Model file for the job. Use its own axes, mm. Round coordinates to 2 decimals unless told otherwise and drop trailing zeros. Order: outer loops, then holes, each group sorted by start corner. A loop starts at its lowest first (then second) coordinate and runs counter-clockwise, first axis right, second up. Notation, with made-up numbers: (80.25, -8.75) - (112.25, -8.75) arc R20 cw to (112.25, 18.25) - close; hole circle Ø2 at (-30, 60.5). An arc over 180 degrees is marked (long way). Write item = value, one per line.
```python
from build123d import *

# Parameters (mm, degrees)
F1_DEPTH = 25.4


with BuildPart() as f1:
    # F0 (on Right) → F1 (new body)
    with BuildSketch(Plane.YZ):
        with BuildLine():
            ThreePointArc((-32.9688712955, -74.7904999055), (-16.4519134228, -59.7619169827), (0.0058700323, -74.8552786289))
            Line((0.0058700323, -74.8552786289), (0.610534451, 75.7063031197))
            Line((0.610534451, 75.7063031197), (-32.9688712955, 75.7063031197))
            Line((-32.9688712955, 75.7063031197), (-32.9688712955, -74.7904999055))
        make_face()
        with BuildLine():
            Line((-9.1503931598, -76.3168334961), (3.395e-07, -76.3168334961))
            Line((3.395e-07, -76.3168334961), (0.0058700323, -74.8552786289))
            ThreePointArc((0.0058700323, -74.8552786289), (-16.4519134228, -59.7619169827), (-32.9688712955, -74.7904999055))
            Line((-32.9688712955, -74.7904999055), (-32.9688712955, -76.3168334961))
            Line((-32.9688712955, -76.3168334961), (-23.8184777961, -76.3168334961))
            ThreePointArc((-23.8184777961, -76.3168334961), (-16.484435478, -68.982791178), (-9.1503931598, -76.3168334961))
        make_face()
        with BuildLine():
            Line((0.0058700323, -74.8552786289), (3.395e-07, -76.3168334961))
            Line((3.395e-07, -76.3168334961), (-9.1503931598, -76.3168334961))
            ThreePointArc((-9.1503931598, -76.3168334961), (-16.484435478, -83.6508758142), (-23.8184777961, -76.3168334961))
            Line((-23.8184777961, -76.3168334961), (-32.9688712955, -76.3168334961))
            Line((-32.9688712955, -76.3168334961), (-32.9688712955, -74.7904999055))
            ThreePointArc((-32.9688712955, -74.7904999055), (-17.2484162143, -92.8541443986), (0.0705129802, -76.3168334961))
            ThreePointArc((0.0705129802, -76.3168334961), (0.0543443475, -75.5853416403), (0.0058700323, -74.8552786289))
        make_face()
    extrude(amount=F1_DEPTH)


solid = f1.part
```
1) Cut at A-A (x = 17.5). Write the cut outline in (y, z).
Conclusion:
outline = (-32.97, -74.79) arc R16.55 ccw (long way) to (0.01, -74.86) - (0.61, 75.71) - (-32.97, 75.71) - close; hole circle Ø14.67 at (-16.48, -76.32)
2) Wall check: line 1 along Z through (x, y) = (20.5, -22.5); line 2 along Y through (x, z) = (5.25, -62.5); line 3 along Y through (x, z) = (16.5, -75). Give the ranges that are in metal, low to high.
Conclusion:
line_1 = -91.74 to -80.51, -72.12 to 75.71
line_2 = -32.97 to 0.06
line_3 = -32.99 to -23.7, -9.27 to 0.02
3) Cut at D-D (y = -1.5). Write the cut outline in (x, z).
Conclusion:
outline = (0, -83.35) - (25.4, -83.35) - (25.4, 75.71) - (0, 75.71) - close
4) Cut at B-B (y = -21.5). Write the cut outline in (x, z), and give its area (3 significant figures).
Conclusion:
outline = (0, -92.09) - (25.4, -92.09) - (25.4, -81.67) - (0, -81.67) - close; (0, -70.97) - (25.4, -70.97) - (25.4, 75.71) - (0, 75.71) - close
area = 3,990 mm^2
5) Cut at C-C (z = -81). Write the cut outline in (x, y), and give its area (3 significant figures).
Conclusion:
outline = (0, -32.36) - (25.4, -32.36) - (25.4, -22.13) - (0, -22.13) - close; (0, -10.84) - (25.4, -10.84) - (25.4, -0.61) - (0, -0.61) - close
area = 520 mm^2
6) Flat gauge pins, fed straight in: pin 1 Ø10 at (x, z) = (18, 11.5) entering from -Y; pin 2 Ø3 at (x, y) = (12.5, -24) entering from -Z. Where does each tip first touch, or does it go through?
Conclusion:
pin_1 = -32.97
pin_2 = -91.74
